The listing builds one solid part. Answer for the finished solid, in the listing's coordinates (mm). Give positions to 0.01 mm unless a question says otherwise; leave off trailing zeros. Order: outer loops, then holes, each group sorted by start corner. A loop starts at its lowest first (then second) coordinate and runs counter-clockwise, first axis right, second up. Notation, with made-up numbers: (34.5, 16.25) - (92.5, 16.25) arc R28 ccw to (92.5, 39.25) - close; hole circle Ø10 at (40.5, -24). An arc over 180 degrees is marked (long way). Write each question's results on one line, items separated by ' | '. Start each with the question number.
1. Section C-C (x = -39) is taken. Give the vertices of the cut face in (y, z) (3 decimals), and give its area (3 significant figures).
2. Section A-A (x = 0) is taken. Give the vertices of the cut face in (y, z) (3 decimals).
3. A flat-ended cylindrical pin translates along its axis: pin 1 (3 mm diameter, centred on x = -2, y = -1, fed in from +Z). Find the tip coordinate at first contact, or state that the pin passes through.
4. Find the intervals of material crossed by L1, parallel to Z at x = 0, y = -1; L2, parallel to Z at x = 50, y = -3; L3, parallel to Z at x = -1, y = 1.5, in increasing order.
from build123d import *

# Parameters (mm, degrees)
SKETCH1_W               = 287.02
SKETCH1_H               = 201.676
BOSS_EXTRUDE1_DEPTH     = 3.175
SKETCH2_W               = 149.225
SKETCH2_H               = 25.4
CUT_EXTRUDE1_DEPTH      = 1
CUT_EXTRUDE1_DEPTH_BACK = 7.35
SKETCH3_R               = 3.175
CUT_EXTRUDE2_DEPTH      = 1
CUT_EXTRUDE2_DEPTH_BACK = 7.35


with BuildPart() as part:
    # Sketch1 → Boss-Extrude1 (new body, symmetric)
    with BuildSketch(Plane(origin=(0, 0, 0), x_dir=(1, 0, 0), z_dir=(0, 1, 0))):
        Rectangle(SKETCH1_W, SKETCH1_H)
    extrude(amount=BOSS_EXTRUDE1_DEPTH, both=True)

    # Sketch2 → Cut-Extrude1 (cut, two sides)
    with BuildSketch(Plane(origin=(0, 3.175, 0), x_dir=(1, 0, 0), z_dir=(0, 1, 0))) as cut_extrude1_sk:
        with Locations((0, -88.138)):
            Rectangle(SKETCH2_W, SKETCH2_H)
    extrude(amount=CUT_EXTRUDE1_DEPTH, mode=Mode.SUBTRACT)
    extrude(cut_extrude1_sk.sketch, amount=-CUT_EXTRUDE1_DEPTH_BACK, mode=Mode.SUBTRACT)

    # Sketch3 → Cut-Extrude2 (cut, two sides)
    with BuildSketch(Plane.XZ.offset(3.175)) as cut_extrude2_sk:
        with Locations((41.91, 88.138)):
            Circle(SKETCH3_R)
        with Locations((0, -84.328)):
            Circle(SKETCH3_R)
        with Locations((-41.91, 88.138)):
            Circle(SKETCH3_R)
    extrude(amount=CUT_EXTRUDE2_DEPTH, mode=Mode.SUBTRACT)
    extrude(cut_extrude2_sk.sketch, amount=-CUT_EXTRUDE2_DEPTH_BACK, mode=Mode.SUBTRACT)


solid = part.part
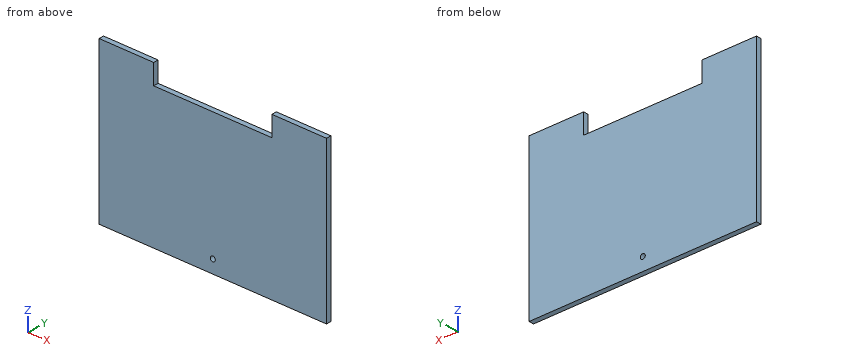
Reported:
1) outline: (-3.175, -100.838) - (3.175, -100.838) - (3.175, 75.438) - (-3.175, 75.438) - close | area: 1,120 mm²
2) outline: (-3.175, -100.838) - (3.175, -100.838) - (3.175, -87.503) - (-3.175, -87.503) - close; (-3.175, -81.153) - (3.175, -81.153) - (3.175, 75.438) - (-3.175, 75.438) - close
3) pin 1: z = 75.44
4) L1: -100.84 to -87.5, -81.15 to 75.44 | L2: -100.84 to 75.44 | L3: -100.84 to -87.34, -81.31 to 75.44
